Autodesk Fusion 360 part; units mm, degrees
sketch "Sketch1" plane through (0, 0, 0) normal (0, 1, 0) x (1, 0, 0)
  line L0 (0, 0) -> (300, 0)
  line L1 (300, 0) -> (300, 400)
  line L2 (300, 400) -> (0, 400)
  line L3 (0, 400) -> (0, 0)
  line L4 (0, 0) -> (10, 0)
  line L5 (0, 0) -> (9.8603, 0)
  line L6 (0, 10) -> (0, 0)
  line L7 (9.8603, 10) -> (289.8603, 10)
  line L8 (289.8603, 10) -> (289.8603, 390)
  line L9 (289.8603, 390) -> (9.8603, 390)
  line L10 (9.8603, 390) -> (9.8603, 10)
extrude "Extrude1" add sketch "Sketch1" along normal blind 10 contours L0 L1 L2 L3 L4 L5 L6 | L7 L8 L9 L10
sketch "Sketch2" plane through (0, 10, 0) normal (0, 1, 0) x (-1, 0, 0)
  line L0 (0, -400) -> (0, 0)
  line L1 (0, 0) -> (-300, 0)
  line L2 (-300, 0) -> (-300, -400)
  line L3 (-300, -400) -> (0, -400)
  line L4 (0, 0) -> (-10, 0)
  line L5 (0, -10) -> (0, 0)
  line L6 (-10, -10) -> (-290, -10)
  line L7 (-290, -10) -> (-290, -390)
  line L8 (-290, -390) -> (-10, -390)
  line L9 (-10, -390) -> (-10, -10)
  line L10 (0, 0) -> (-300, 0)
  line L11 (-300, 0) -> (-300, -400)
  line L12 (-300, -400) -> (0, -400)
  line L13 (0, -400) -> (0, 0)
extrude "Extrude2" add sketch "Sketch2" along normal blind 100
Geometry: final body of the model. Coordinates: model frame, mm. A direction names the side the tool comes from. Give positions to 0.01 mm unless a question says otherwise; leave off trailing zeros. Write each loop counter-clockwise with the first axis right and the second up, starting at its lowest first coordinate (ties: lowest second). Pieces come first, ordered by that corner, then holes.
(1) Mould query, pull axis X, two halves, no side actions, for faces 3 (the flat face through (152, 59, -390)), 4 (the flat face through (148, 0, -203)), 5 (the flat face through (300, 54, -197)). Classes: released by +X, released by -X, zero draft, split by the parting line, or undercut.
(2) Access query for faces 1 (the flat face through (148, 54, 0)), 2 (the flat face through (10, 59, -203)). Directions: +Z, -Z, +X, -X, +Y, -Y. A direction counts if a zero-diameter tool reaches every point of the face in a straight line with its end or side. Return the directions, or none.
(3) Cut plane B-B, the plane z = -148.5. Return loops of the section in (x, y).
(4) Ray query, line 1 (Z direction, x = 148, y = 46); line 2 (X direction, y = 81, z = -364.5); line 3 (Y direction, x = 288.5, z = -276). Return the intervals inside material, ascending.
(5) Cut plane C-C, the plane x = 23. Return loops of the section in (y, z), then the cut area to 3 significant figures.
(6) Cut plane A-A, the plane y = 60. Return loops of the section in (x, z), then the cut area to 3 significant figures.
Values follow:
1. face 3: undercut
1. face 4: zero draft
1. face 5: released by +X
2. face 1: +Z, +X, -X, +Y, -Y
2. face 2: +Y
3. outline: (0, 0) - (300, 0) - (300, 110) - (290, 110) - (290, 10) - (10, 10) - (10, 110) - (0, 110) - close
4. line 1: z = -400 to -390, -10 to 0
4. line 2: x = 0 to 10, 290 to 300
4. line 3: y = 0 to 10
5. outline: (0, -400) - (110, -400) - (110, -390) - (10, -390) - (10, -10) - (110, -10) - (110, 0) - (0, 0) - close
5. area: 6,000 mm2
6. outline: (0, -400) - (300, -400) - (300, 0) - (0, 0) - close; hole (10, -390) - (290, -390) - (290, -10) - (10, -10) - close
6. area: 13,600 mm2
